```python
from build123d import *

# Parameters (mm, degrees)
CROQUIS1_W              = 25
CROQUIS1_H              = 12.5
SALIENTE_EXTRUIR2_DEPTH = 16
CORTAR_EXTRUIR3_START   = -3.5
CROQUIS2_R              = 12.5
CROQUIS2_R_2            = 5
CORTAR_EXTRUIR3_DEPTH   = 3.5
REDONDEO5_R             = 5
REDONDEO6_R             = 5
SALIENTE_EXTRUIR3_DEPTH = 3.5
CHAFL_N1_SIZE           = 1
CHAFL_N2_SIZE           = 1
CHAFL_N3_SIZE           = 1
CHAFL_N4_SIZE           = 1
CHAFL_N5_SIZE           = 1
CHAFL_N6_SIZE           = 1
CORTAR_EXTRUIR5_DEPTH   = 10
REDONDEO9_R             = 5
REDONDEO10_R            = 5
CROQUIS5_R              = 2.5
CORTAR_EXTRUIR6_DEPTH   = 5
CORTAR_EXTRUIR9_START   = -3.5
CORTAR_EXTRUIR9_DEPTH   = 3.5
REDONDEO12_START        = 12.5
REDONDEO12_DEPTH        = 4.5


with BuildPart() as part:
    # Croquis1 → Saliente-Extruir2 (new body)
    with BuildSketch(Plane.XY):
        with Locations((0, 36.25)):
            Rectangle(CROQUIS1_W, CROQUIS1_H)
        with Locations((0, 23.75)):
            Rectangle(CROQUIS1_W, CROQUIS1_H)
        with BuildLine():
            Line((-12.5, 17.5), (-12.5, -30))
            ThreePointArc((-12.5, -30), (0, -17.5), (12.5, -30))
            Line((12.5, -30), (12.5, 17.5))
            Line((12.5, 17.5), (-12.5, 17.5))
        make_face()
        with BuildLine():
            ThreePointArc((12.5, -30), (0, -17.5), (-12.5, -30))
            Line((-12.5, -30), (12.5, -30))
        make_face()
        with BuildLine():
            Line((12.5, -30), (-12.5, -30))
            ThreePointArc((-12.5, -30), (0, -42.5), (12.5, -30))
        make_face()
    extrude(amount=SALIENTE_EXTRUIR2_DEPTH)

    # Croquis2 → Cortar-Extruir3 (cut)
    with BuildSketch(Plane.XY.offset(16).offset(CORTAR_EXTRUIR3_START)):
        with Locations((0, -30)):
            Circle(CROQUIS2_R)
        with Locations((0, -30)):
            Circle(CROQUIS2_R_2, mode=Mode.SUBTRACT)
    extrude(amount=CORTAR_EXTRUIR3_DEPTH, mode=Mode.SUBTRACT)

    # Redondeo5
    redondeo5_edges = [part.edges().sort_by_distance(p)[0] for p in [
        (-12.5, -30, 14.25),
    ]]
    fillet(redondeo5_edges, radius=REDONDEO5_R)

    # Redondeo6
    redondeo6_edges = [part.edges().sort_by_distance(p)[0] for p in [
        (12.5, -30, 14.25),
    ]]
    fillet(redondeo6_edges, radius=REDONDEO6_R)

    # Croquis3 → Saliente-Extruir3 (add)
    with BuildSketch(Plane.XY.offset(16)):
        Polygon((6.92820323, -30), (3.464101615, -24), (-3.464101615, -24), (-6.92820323, -30), (-3.464101615, -36), (3.464101615, -36), align=None)
    extrude(amount=SALIENTE_EXTRUIR3_DEPTH)

    # Chaflán1
    chafl_n1_edges = [part.edges().sort_by_distance(p)[0] for p in [
        (5.196152423, -27, 19.5),
    ]]
    chamfer(chafl_n1_edges, length=CHAFL_N1_SIZE)

    # Chaflán2
    chafl_n2_edges = [part.edges().sort_by_distance(p)[0] for p in [
        (-0.577350269, -24, 19.5),
    ]]
    chamfer(chafl_n2_edges, length=CHAFL_N2_SIZE)

    # Chaflán3
    chafl_n3_edges = [part.edges().sort_by_distance(p)[0] for p in [
        (4.907477288, -33.5, 19.5),
    ]]
    chamfer(chafl_n3_edges, length=CHAFL_N3_SIZE)

    # Chaflán4
    chafl_n4_edges = [part.edges().sort_by_distance(p)[0] for p in [
        (-0.577350269, -36, 19.5),
    ]]
    chamfer(chafl_n4_edges, length=CHAFL_N4_SIZE)

    # Chaflán5
    chafl_n5_edges = [part.edges().sort_by_distance(p)[0] for p in [
        (-5.484827557, -32.5, 19.5),
    ]]
    chamfer(chafl_n5_edges, length=CHAFL_N5_SIZE)

    # Chaflán6
    chafl_n6_edges = [part.edges().sort_by_distance(p)[0] for p in [
        (-5.196152423, -27, 19.5),
    ]]
    chamfer(chafl_n6_edges, length=CHAFL_N6_SIZE)

    # Croquis4 → Cortar-Extruir5 (cut)
    with BuildSketch(Plane(origin=(0, 42.5, 0), x_dir=(1, 0, 0), z_dir=(0, 1, 0))):
        with BuildLine():
            ThreePointArc((-8, -8), (-5.656854249, -2.343145751), (0, 0))
            Line((0, 0), (-12.5, 0))
            Line((-12.5, 0), (-12.5, -8))
            Line((-12.5, -8), (-8, -8))
        make_face()
        with BuildLine():
            ThreePointArc((0, -16), (-5.656854249, -13.656854249), (-8, -8))
            Line((-8, -8), (-12.5, -8))
            Line((-12.5, -8), (-12.5, -16))
            Line((-12.5, -16), (0, -16))
        make_face()
        with BuildLine():
            Line((12.5, -8), (8, -8))
            ThreePointArc((8, -8), (5.656854249, -13.656854249), (0, -16))
            Line((0, -16), (12.5, -16))
            Line((12.5, -16), (12.5, -8))
        make_face()
        with BuildLine():
            Line((12.5, 0), (0, 0))
            ThreePointArc((0, 0), (5.656854249, -2.343145751), (8, -8))
            Line((8, -8), (12.5, -8))
            Line((12.5, -8), (12.5, 0))
        make_face()
    extrude(amount=-CORTAR_EXTRUIR5_DEPTH, mode=Mode.SUBTRACT)

    # Redondeo9
    redondeo9_edges = [part.edges().sort_by_distance(p)[0] for p in [
        (12.5, 32.5, 8),
    ]]
    fillet(redondeo9_edges, radius=REDONDEO9_R)

    # Redondeo10
    redondeo10_edges = [part.edges().sort_by_distance(p)[0] for p in [
        (-12.5, 32.5, 8),
    ]]
    fillet(redondeo10_edges, radius=REDONDEO10_R)

    # Croquis5 → Cortar-Extruir6 (cut)
    with BuildSketch(Plane(origin=(0, 42.5, 0), x_dir=(1, 0, 0), z_dir=(0, 1, 0))):
        with Locations(Location((0, -8, 0), (0, 0, 270))):
            Circle(CROQUIS5_R)
    extrude(amount=-CORTAR_EXTRUIR6_DEPTH, mode=Mode.SUBTRACT)

    # Chaflán7: read off the stored shape, not the designer's step
    # Chaflán7 outline → Chaflán7 (revolve, cut)
    with BuildSketch(Plane.XY.offset(8)):
        Polygon((8, 42.5), (7, 42.5), (8, 41.5), align=None)
    revolve(axis=Axis((0, 0, 8), (0, 1, 0)), mode=Mode.SUBTRACT)

    # Croquis7 → Cortar-Extruir9 (cut)
    with BuildSketch(Plane.XY.offset(16).offset(CORTAR_EXTRUIR9_START)):
        with BuildLine():
            Line((-12.5, 27.5), (5.357142857, -18.706151214))
            ThreePointArc((5.357142857, -18.706151214), (0, -17.5), (-5.357142857, -18.706151214))
            ThreePointArc((-5.357142857, -18.706151214), (-10.172612419, -18.414382973), (-12.5, -14.188611699))
            Line((-12.5, -14.188611699), (-12.5, 27.5))
        make_face()
    extrude(amount=CORTAR_EXTRUIR9_DEPTH, mode=Mode.SUBTRACT)

    # Redondeo12: read off the stored shape, not the designer's step
    # Redondeo12 outline → Redondeo12 (cut)
    with BuildSketch(Plane.XY.offset(REDONDEO12_START)):
        with BuildLine():
            ThreePointArc((12.5, -10.380609645), (8.416748435, -15.29584843), (2.836171077, -12.18302463))
            Line((2.836171077, -12.18302463), (5.357142857, -18.706151214))
            ThreePointArc((5.357142857, -18.706151214), (10.172612419, -18.414382973), (12.5, -14.188611699))
            Line((12.5, -14.188611699), (12.5, -10.380609645))
        make_face()
    extrude(amount=REDONDEO12_DEPTH, mode=Mode.SUBTRACT)


solid = part.part
```
Check sheet for the modelled part. Datum: model origin and axes. Units: mm. A direction names the side the tool comes from. Round coordinates to 2 decimals unless told otherwise and drop trailing zeros. Loops run counter-clockwise (first coordinate to the right, second up) from the corner with the lowest first, then second, coordinate; pieces in that order, holes last. Notation, with made-up numbers: (-5.75, 13) -> (32.25, 13) arc R24 cw to (32.25, 37) -> close; hole circle Ø11 at (-23.5, 46.5). An arc over 180 degrees is marked (long way). Answer in a Markdown table with one row per item.
Q1. Go/stop test with flat-tipped pins: P1, Ø1, axis at x = 4, z = 14.5, coming from the -Y side; P2, Ø4, axis at x = 8, y = 3.5, coming from the +Z side; P3, Ø2, axis at x = -1.5, z = 17.5, coming from the +Y side. Record where each tip stops, or that it passes through.
Data:
| item | result |
|---|---|
| P1 | stops at y = -33.57 |
| P2 | stops at z = 16 |
| P3 | stops at y = -24 |
Q2. Sectioned sample at A-A on y = 1. Enter the section's corners in (x, z).
Data:
| item | result |
|---|---|
| outline | (-12.5, 0) -> (12.5, 0) -> (12.5, 16) -> (-2.26, 16) -> (-2.26, 12.5) -> (-12.5, 12.5) -> close |
Q3. Thickness scan on L1, parallel to X at y = 39.95, z = 8; L2, parallel to Z at x = -9.5, y = -0.5; L3, parallel to Z at x = -0.25, y = 15. Record the ranges inside material, lowest first.
Data:
| item | result |
|---|---|
| L1 | x = -8 to -2.5, 2.5 to 8 |
| L2 | z = 0 to 12.5 |
| L3 | z = 0 to 16 |
Q4. Release check for a two-part mould opening along Y. For faces 4 (the face through (12.5, -2, 8)), 5 (the face through (2, -25, 16)), 6 (the face through (-11, 31.07, 13.43)) record: released by +Y, released by -Y, zero draft, split by the parting line, or undercut.
Data:
| item | result |
|---|---|
| face 4 | zero draft |
| face 5 | undercut |
| face 6 | released by +Y |
Q5. Set-up check for faces 1 (the face through (-11, 31.07, 2.64)), 2 (the face through (-5.172, -26.958, 17.232)), 3 (the face through (-5.22, -32.96, 17.23)): record each of +Z, -Z, +X, -X, +Y, -Y from which the full face is reachable in a straight line by a thin tool's end or side.
Data:
| item | result |
|---|---|
| face 1 | -Z, -X, +Y |
| face 2 | +Z, -X, +Y |
| face 3 | +Z, -X, -Y |
